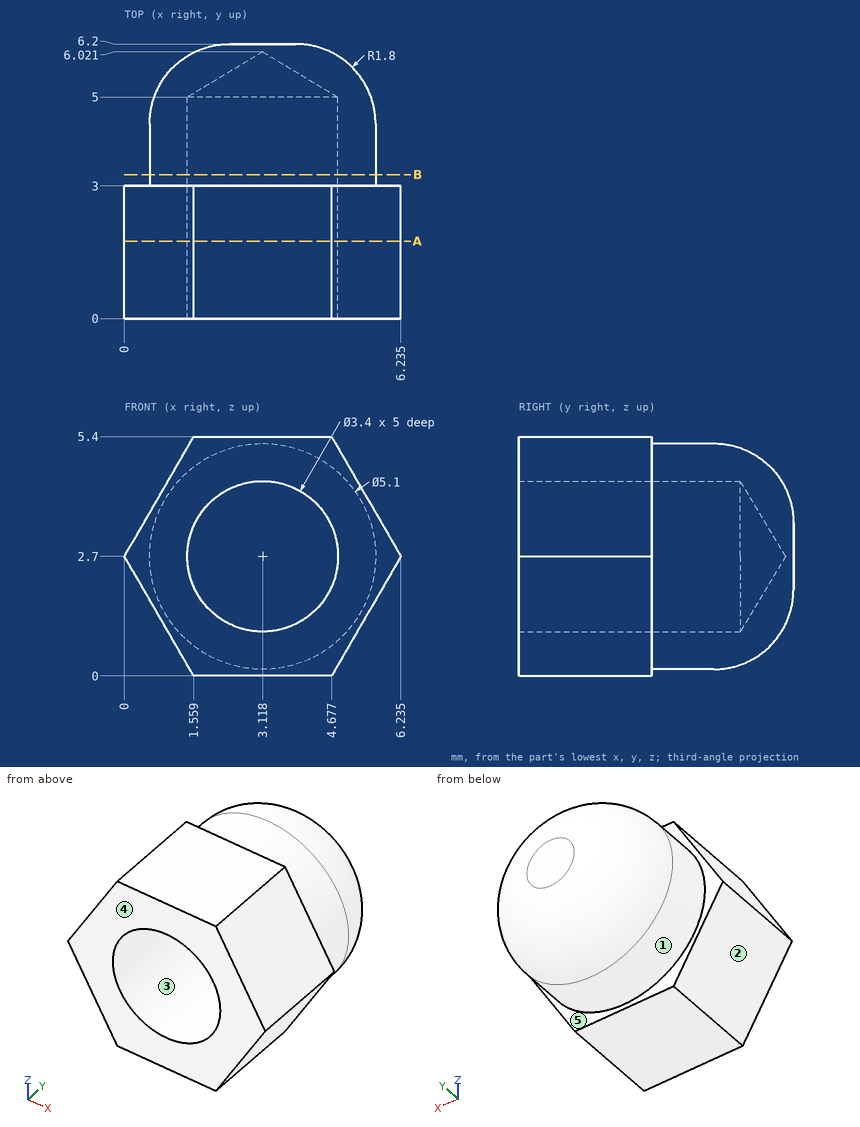
Verification items for this drawing (mm, ordinates from the low corner). A direction names the side the tool comes from. Give positions to 0.01 mm unless a question says otherwise; leave off trailing zeros. Loops run counter-clockwise (first coordinate to the right, second up) from the corner with the lowest first, then second, coordinate; pieces in that order, holes last. Notation, with made-up numbers: M -24,38.5 L -6,38.5 A14 ccw -6,56.5 Z; hole C 64,34 d2. An arc over 180 degrees is marked long. Write item = value, one per line.
(1) Material ranges on line 1 (X direction, y = 3.5, z = 3.35) (1 decimal); line 2 (X direction, y = 3.25, z = 1.8) (1 decimal); line 3 (Z direction, x = 2.25, y = 1), recorded low to high. Write a range as [from, to].
Answer below:
line_1 = [0.7, 1.5], [4.7, 5.6]
line_2 = [0.7, 1.7], [4.6, 5.5]
line_3 = [0, 1.24], [4.16, 5.4]
(2) Tool access check on the marked faces 4 and 5. Record the directions out of +Z, -Z, +X, -X, +Y, -Y that give a thin tool (end or side, any length) a straight path to the whole face; none if there is none.
Answer below:
face_4 = +Z, -Z, +X, -X, -Y
face_5 = +Y
(3) Gauge pin test, flat ends, axial feed: pin 1 Ø1.5 at (x, y) = (5.5, 3) entering from +Z (1 decimal); pin 2 Ø1 at (x, z) = (2, 3.5) entering from +Y. Record the tip position at first contact, or that the pin passes through.
Answer below:
pin_1 = 5.3
pin_2 = 6.2
(4) Sectioned sample at A-A, the plane y = 1.75. Record the cut outline in (x, z) (1 decimal).
Answer below:
outline = M 0,2.7 L 1.6,0 L 4.7,0 L 6.2,2.7 L 4.7,5.4 L 1.6,5.4 Z; hole C 3.1,2.7 d3.4
(5) Sectioned sample at B-B, the plane y = 3.25. Record the cut outline in (x, z).
Answer below:
outline = C 3.12,2.7 d5.1; hole C 3.12,2.7 d3.4
(6) Release check for a two-part mould opening along X. For the marked faces 1, 2 and 3 record: released by +X, released by -X, zero draft, split by the parting line, or undercut.
Answer below:
face_1 = split by the parting line
face_2 = released by -X
face_3 = undercut
